The listing builds one solid part. Answer for the finished solid, in the listing's coordinates (mm). A direction names the side the tool comes from. Coordinates: 2 decimals unless noted, no trailing zeros. Order: outer loops, then holes, each group sorted by start corner. A loop starts at its lowest first (then second) coordinate and runs counter-clockwise, first axis right, second up. Notation, with made-up numbers: (37.25, 54.5) -> (64.25, 54.5) arc R30 cw to (64.25, 79.5) -> close; hole circle Ø8 at (50.25, 39.5). An arc over 180 degrees is marked (long way). Answer in a Markdown table with one row per item. Add a question column.
Autodesk Inventor part; units mm, degrees
ref_plane "YZ Plane" through (0, 0, 0) normal (1, 0, 0) x (0, 1, 0)
ref_plane "XZ Plane" through (0, 0, 0) normal (0, 1, 0) x (-1, 0, 0)
ref_plane "XY Plane" through (0, 0, 0) normal (0, 0, 1) x (1, 0, 0)
sketch "Sketch1" plane through (0, 0, 0) normal (0, 1, 0) x (-1, 0, 0)
  line L0 (50, 50) -> (-50, 50)
  line L1 (-50, 50) -> (-50, -50)
  line L2 (-50, -50) -> (50, -50)
  line L3 (50, -50) -> (50, 50)
  line L4 (-50, 50) -> (50, -50) construction
  line L5 (-47.5, 47.5) -> (47.5, 47.5)
  line L6 (47.5, 47.5) -> (47.5, -47.5)
  line L7 (47.5, -47.5) -> (-47.5, -47.5)
  line L8 (-47.5, -47.5) -> (-47.5, 47.5)
  line L9 (-47.5, 47.5) -> (47.5, -47.5) construction
  circle A0 centre (0, 0) radius 22.5
  circle A1 centre (0, 0) radius 15
  line L10 (40.4289, 47.5) -> (11.9766, 19.0476)
  line L11 (47.5, 40.4289) -> (19.0476, 11.9765)
  line L12 (-47.5, 40.4289) -> (-19.0476, 11.9766)
  line L13 (-40.4289, 47.5) -> (-11.9765, 19.0476)
  line L14 (-40.4289, -47.5) -> (-11.9766, -19.0476)
  line L15 (-47.5, -40.4289) -> (-19.0476, -11.9765)
  line L16 (47.5, -40.4289) -> (19.0476, -11.9766)
  line L17 (40.4289, -47.5) -> (11.9765, -19.0476)
  circle A2 centre (35, -35) radius 2
  circle A3 centre (35, 35) radius 2
  circle A4 centre (-35, 35) radius 2
  circle A5 centre (-35, -35) radius 2
  point P0 (19.0476, -11.9766)
  point P1 (-11.9765, 19.0476)
  point P2 (-11.9766, -19.0476)
  point P3 (11.9765, -19.0476)
  dimension "d0" = 100
  dimension "d1" = 100
  dimension "d2" = 95
  dimension "d3" = 95
  dimension "d9" = 30
  dimension "d10" = 7.5
  dimension "d11" = 10
  dimension "d12" = 7.0711
  dimension "d13" = 7.0711
  dimension "d16" = 360
  dimension "d23" = 4
  dimension "d24" = 35
  dimension "d27" = 360
extrude "Extrusion1" add sketch "Sketch1" along normal blind 10 contours L3 L2 L1 L0 | L5 L13 A0 L12 L8 | L5 L6 L11 A0 L10 | A0 | L15 A0 L14 L7 L8 | L6 L7 L17 A0 L16 | A2 | A3 | A4 | A5
sketch "Sketch3" plane through (0, 10, 0) normal (0, 1, 0) x (1, 0, 0)
  line L0 (-50, -50) -> (-40.43, -50)
  line L1 (-40.43, -50) -> (-40.43, -40.43)
  line L2 (-40.43, -40.43) -> (-50, -40.43)
  line L3 (-50, -40.43) -> (-50, -50)
  line L4 (40.43, -40.43) -> (40.43, -50)
  line L5 (40.43, -50) -> (50, -50)
  line L6 (50, -40.43) -> (40.43, -40.43)
  line L7 (50, -50) -> (50, -40.43)
  line L8 (40.43, 40.43) -> (50, 40.43)
  line L9 (50, 40.43) -> (50, 50)
  line L10 (40.43, 50) -> (40.43, 40.43)
  line L11 (50, 50) -> (40.43, 50)
  line L12 (-40.43, 40.43) -> (-40.43, 50)
  line L13 (-40.43, 50) -> (-50, 50)
  line L14 (-50, 40.43) -> (-40.43, 40.43)
  line L15 (-50, 50) -> (-50, 40.43)
  point P0 (0, 0)
  dimension "d29" = 9.57
  dimension "d30" = 9.57
  dimension "d33" = 360
extrude "Extrusion2" add sketch "Sketch3" along normal blind 6.75
sketch "Sketch4" plane through (-50, 0, -50) normal (-1, 0, 0) x (0, 0, 1)
  circle A0 centre (30, 5) radius 2
  line L0 (0, 0) -> (0, 16.75)
  circle A1 centre (70, 5) radius 2
  line L1 (100, 0) -> (100, 16.75)
  point P0 (50, 0)
  dimension "d37" = 4
  dimension "d38" = 30
  dimension "d39" = 4
  dimension "d40" = 30
extrude "Extrusion3" cut sketch "Sketch4" against normal blind 6.75
sketch "Sketch5" plane through (50, 0, 50) normal (1, 0, 0) x (0, 0, -1)
  circle A0 centre (30, 5) radius 2
  line L0 (0, 0) -> (0, 16.75)
  circle A1 centre (70, 5) radius 2
  line L1 (100, 0) -> (100, 16.75)
  point P0 (50, 0)
  dimension "d43" = 4
  dimension "d44" = 30
  dimension "d45" = 4
  dimension "d46" = 30
extrude "Extrusion4" cut sketch "Sketch5" against normal blind 6.75
sketch "Sketch6" plane through (0, 0, 0) normal (0, -1, 0) x (1, 0, 0)
  line L0 (35, 45) -> (-35, 45)
  line L1 (-35, 45) -> (-35, -45)
  line L2 (-35, -45) -> (35, -45)
  line L3 (35, -45) -> (35, 45)
  line L4 (35, 45) -> (-35, -45) construction
  line L5 (-35, 45) -> (35, -45) construction
  line L6 (40.4289, 47.5) -> (25.4289, 47.5)
  line L7 (40.4289, 47.5) -> (-40.4289, 47.5)
  line L8 (25.4289, 47.5) -> (25.4289, 32.5)
  line L9 (25.4289, 32.5) -> (40.4289, 47.5)
  line L10 (40.4289, -47.5) -> (11.9766, -19.0476)
  line L11 (40.4289, -47.5) -> (25.4289, -47.5)
  line L12 (-40.4289, -47.5) -> (40.4289, -47.5)
  line L13 (-40.4289, 47.5) -> (-25.4289, 47.5)
  line L14 (-40.4289, -47.5) -> (-25.4289, -47.5)
  circle A0 centre (32.5, 42) radius 1.5
  circle A1 centre (32.5, -42) radius 1.5
  circle A2 centre (-33, -42) radius 1.5
  circle A3 centre (-33, 42) radius 1.5
  line L15 (-40.4289, -47.5) -> (-25.4289, -47.5)
  line L16 (-25.4289, -47.5) -> (-25.4289, -32.5)
  line L17 (-25.4289, -32.5) -> (-40.4289, -47.5)
  line L18 (-40.4289, 47.5) -> (-25.4289, 47.5)
  line L19 (-40.4289, 47.5) -> (-25.4289, 47.5)
  line L20 (-40.4289, 47.5) -> (-25.4289, 47.5) construction
  line L21 (-25.4289, 47.5) -> (-25.4289, 32.5)
  line L22 (-25.4289, 32.5) -> (-40.4289, 47.5)
  line L23 (25.4289, -47.5) -> (25.4289, -32.5)
  line L24 (25.4289, -47.5) -> (40.4289, -47.5) construction
  line L25 (25.4289, -32.5) -> (40.4289, -47.5)
  point P0 (0, 0)
  point P1 (-34.4058, -41.4769)
  point P2 (-33.5231, -40.5942)
  point P3 (-33.5231, 40.5942)
  point P4 (-34.4058, 41.4769)
  dimension "d49" = 70
  dimension "d50" = 90
  dimension "d51" = 15
  dimension "d52" = 15
  dimension "d53" = 90
  dimension "d54" = 15
  dimension "d56" = 15
  dimension "d58" = 15
  dimension "d59" = 3
  dimension "d60" = 2.5
  dimension "d61" = 3
  dimension "d62" = 3
  dimension "d63" = 3
  dimension "d64" = 2.5
  dimension "d65" = 3
  dimension "d66" = 3
  dimension "d67" = 2
  dimension "d68" = 3
  dimension "d69" = 3
  dimension "d70" = 2
  dimension "d71" = 15
  dimension "d72" = 15
  dimension "d73" = 0
  dimension "d74" = 15
  dimension "d75" = 90
  dimension "d76" = 15
  dimension "d77" = 90
extrude "Extrusion5" cut sketch "Sketch6" against normal blind 10 contours A3 L22 | A2 L17 picked at (-33.9131, 40.9363) picked at (-33.9131, -40.9363)
extrude "Extrusion6" add sketch "Sketch6" against normal blind 10 contours L3 L9 L8 L0 | L0 L8 L6 L9 L3 | L21 L22 A3 L1 L0 | L0 L1 L22 L7 L21 | L10 L11 L23 L2 L3 | L3 L2 L23 L10 | L17 A2 L16 L2 L1 | L1 L2 L16 L12 L17
sketch "Sketch8" plane through (0, 10, 0) normal (0, 1, 0) x (1, 0, 0)
  circle A0 centre (-33, 42) radius 1.5
  circle A1 centre (-33, 42) radius 1.5
  circle A2 centre (32.5, 42) radius 1.5
  circle A3 centre (32.5, 42) radius 1.5
  circle A4 centre (32.5, -42) radius 1.5
  circle A5 centre (32.5, -42) radius 1.5
  circle A6 centre (-33, -42) radius 1.5
  point P0 (0, 0)
extrude "Extrusion7" add sketch "Sketch8" against normal blind 4
equation "\"d18\" = d11"
properties part number "Top&Bottom"
Q1. A cutting plane is placed at C-C (x = 32.5). Determine the outline of the cut face in (y, z), then the cut area to 3 significant figures.
Q2. Straight lines are drawn through the part: line 1 (X direction, y = 4.65, z = 42); line 2 (Y direction, x = 48.25, z = -20); line 3 (Z direction, x = -33, y = 1.7). For each, find the intervals that lie inside material, in ascending order.
Q3. Given pin 1 (1.5 mm diameter, centred on x = 32.5, z = 42, fed in from -Y); pin 2 (2.5 mm diameter, centred on y = 5, z = 20, fed in from +X); pin 3 (3.5 mm diameter, centred on x = 32.5, z = 42, fed in from +Y), each flat-ended and moving along its own axis, determine where each tip first touches the part or whether it passes through.
Q4. A cutting plane is placed at A-A (y = 12.25). Determine the outline of the cut face in (x, z).
Q5. For faces 1 (the face through (-50, 6, -1)), 2 (the face through (-45, 13, 40.43)), 3 (the face through (-33, 6, 42)), 4 (the face through (-49, 5, 18)), 5 (the face through (18.8, 4.93, -25.87)), determine the directions among +Z, -Z, +X, -X, +Y, -Y from which every point of the face is accessible in a straight line to the end or side of a thin tool.
Q6. A cutting plane is placed at D-D (x = 20.5). Determine the outline of the cut face in (y, z).
Q7. A cutting plane is placed at B-B (x = 0). Determine the outline of the cut face in (y, z).
Q8. Determine the mould class of faces 6 (the face through (45, 16.75, 45)), 7 (the face through (1, 6, -50)), 8 (the face through (18.8, 4.93, 25.87)) for opening direction Z: +Z half, -Z half, draft (parallel to the pull), parting line (faces both ways), or undercut.
Returned:
| question | item | result |
|---|---|---|
| 1 | outline | (0, -50) -> (10, -50) -> (10, -25.43) -> (0, -25.43) -> (0, -40.5) -> (6, -40.5) -> (6, -43.5) -> (0, -43.5) -> close; (0, 25.43) -> (10, 25.43) -> (10, 50) -> (0, 50) -> (0, 43.5) -> (6, 43.5) -> (6, 40.5) -> (0, 40.5) -> close |
| 1 | area | 455 mm² |
| 2 | line 1 | x = -50 to -34.5, -31.5 to -25.43, 25.43 to 31, 34 to 50 |
| 2 | line 2 | y = 0 to 3, 7 to 10 |
| 2 | line 3 | z = -50 to -43.5, -40.5 to -25.93, 25.93 to 40.5, 43.5 to 50 |
| 3 | pin 1 | stops at y = 6 |
| 3 | pin 2 | stops at x = 28.32 |
| 3 | pin 3 | stops at y = 10 |
| 4 | outline | (-50, -50) -> (-40.43, -50) -> (-40.43, -40.43) -> (-50, -40.43) -> close; (-50, 40.43) -> (-40.43, 40.43) -> (-40.43, 50) -> (-50, 50) -> close; (40.43, -50) -> (50, -50) -> (50, -40.43) -> (40.43, -40.43) -> close; (40.43, 40.43) -> (50, 40.43) -> (50, 50) -> (40.43, 50) -> close |
| 5 | face 1 | +Z, -Z, -X, +Y, -Y |
| 5 | face 2 | +X, -X, +Y |
| 5 | face 3 | -Y |
| 5 | face 4 | -X |
| 5 | face 5 | +Y, -Y |
| 6 | outline | (0, -50) -> (10, -50) -> (10, -47.5) -> (0, -47.5) -> close; (0, -27.57) -> (10, -27.57) -> (10, -13.43) -> (0, -13.43) -> close; (0, -9.27) -> (10, -9.27) -> (10, 9.27) -> (0, 9.27) -> close; (0, 13.43) -> (10, 13.43) -> (10, 27.57) -> (0, 27.57) -> close; (0, 47.5) -> (10, 47.5) -> (10, 50) -> (0, 50) -> close |
| 7 | outline | (0, -50) -> (10, -50) -> (10, -47.5) -> (0, -47.5) -> close; (0, -22.5) -> (10, -22.5) -> (10, -15) -> (0, -15) -> close; (0, 15) -> (10, 15) -> (10, 22.5) -> (0, 22.5) -> close; (0, 47.5) -> (10, 47.5) -> (10, 50) -> (0, 50) -> close |
| 8 | face 6 | draft |
| 8 | face 7 | -Z half |
| 8 | face 8 | undercut |
